from build123d import *

# Parameters (mm, degrees)
SKETCH2_R           = 0.75
BOSS_EXTRUDE1_DEPTH = 0.75
SKETCH3_R           = 0.375
BOSS_EXTRUDE2_DEPTH = 0.25
SKETCH4_R           = 1.125
CUT_EXTRUDE1_DEPTH  = 0.15
SKETCH5_R           = 1.1
SKETCH5_R_2         = 0.575
BOSS_EXTRUDE3_DEPTH = 0.15
SKETCH6_R           = 0.375
BOSS_EXTRUDE4_DEPTH = 0.25
SKETCH7_R           = 1.25
CUT_EXTRUDE2_DEPTH  = 5


with BuildPart() as part:
    # Sketch1 → Revolve1 (revolve)
    with BuildSketch(Plane.XY, mode=Mode.PRIVATE) as revolve1_sk:
        Polygon((0, 9.375), (-6.807, 9.375), (-6.807, 8.5), (-5.307, 8.5), (-5.307, 8.125), (-2.907, 8.125), (-2.907, 4.5), (-3.807, 4.5), (-3.807, 3.25), (-4.557, 3.25), (-4.557, 0), (4.557, 0), (4.557, 3.625), (4.057, 3.625), (4.057, 5), (0.943, 5), (0.943, 8.125), (4.193, 8.125), (4.193, 9), (6.193, 9), (6.193, 10), (6.693, 10), (6.693, 10.5), (5.593, 10.5), (5.593, 9.375), align=None)
    revolve(revolve1_sk.sketch.rotate(Axis((-4.557, 0, 0), (1, 0, 0)), 180), axis=Axis((-4.557, 0, 0), (1, 0, 0)))

    # Sketch2 → Boss-Extrude1 (add)
    with BuildSketch(Plane(origin=(0.943, 0, 0), x_dir=(0, 0, -1), z_dir=(1, 0, 0))):
        with Locations(Location((0, 6.25, 0), (0, 0, 270))):
            Circle(SKETCH2_R)
        with Locations(Location((3.125, 5.412658774, 0), (0, 0, 270))):
            Circle(SKETCH2_R)
        with Locations(Location((5.412658774, 3.125, 0), (0, 0, 270))):
            Circle(SKETCH2_R)
        with Locations(Location((6.25, 0, 0), (0, 0, 270))):
            Circle(SKETCH2_R)
        with Locations(Location((5.412658774, -3.125, 0), (0, 0, 270))):
            Circle(SKETCH2_R)
        with Locations(Location((3.125, -5.412658774, 0), (0, 0, 270))):
            Circle(SKETCH2_R)
        with Locations(Location((0, -6.25, 0), (0, 0, 270))):
            Circle(SKETCH2_R)
        with Locations(Location((-3.125, -5.412658774, 0), (0, 0, 270))):
            Circle(SKETCH2_R)
        with Locations(Location((-5.412658774, -3.125, 0), (0, 0, 270))):
            Circle(SKETCH2_R)
        with Locations(Location((-6.25, 0, 0), (0, 0, 270))):
            Circle(SKETCH2_R)
        with Locations(Location((-5.412658774, 3.125, 0), (0, 0, 270))):
            Circle(SKETCH2_R)
        with Locations(Location((-3.125, 5.412658774, 0), (0, 0, 270))):
            Circle(SKETCH2_R)
    extrude(amount=BOSS_EXTRUDE1_DEPTH)

    # Sketch3 → Boss-Extrude2 (add)
    with BuildSketch(Plane(origin=(4.057, 0, 0), x_dir=(0, 0, -1), z_dir=(1, 0, 0))):
        with Locations(Location((0, 4.25, 0), (0, 0, 270))):
            Circle(SKETCH3_R)
        with Locations(Location((2.125, 3.680607966, 0), (0, 0, 270))):
            Circle(SKETCH3_R)
        with Locations(Location((3.680607966, 2.125, 0), (0, 0, 270))):
            Circle(SKETCH3_R)
        with Locations(Location((4.25, 0, 0), (0, 0, 270))):
            Circle(SKETCH3_R)
        with Locations(Location((3.680607966, -2.125, 0), (0, 0, 270))):
            Circle(SKETCH3_R)
        with Locations(Location((2.125, -3.680607966, 0), (0, 0, 270))):
            Circle(SKETCH3_R)
        with Locations(Location((0, -4.25, 0), (0, 0, 270))):
            Circle(SKETCH3_R)
        with Locations(Location((-2.125, -3.680607966, 0), (0, 0, 270))):
            Circle(SKETCH3_R)
        with Locations(Location((-3.680607966, -2.125, 0), (0, 0, 270))):
            Circle(SKETCH3_R)
        with Locations(Location((-4.25, 0, 0), (0, 0, 270))):
            Circle(SKETCH3_R)
        with Locations(Location((-3.680607966, 2.125, 0), (0, 0, 270))):
            Circle(SKETCH3_R)
        with Locations(Location((-2.125, 3.680607966, 0), (0, 0, 270))):
            Circle(SKETCH3_R)
    extrude(amount=BOSS_EXTRUDE2_DEPTH)

    # Sketch4 → Cut-Extrude1 (cut)
    with BuildSketch(Plane(origin=(4.557, 0, 0), x_dir=(0, 0, -1), z_dir=(1, 0, 0))):
        with Locations(Location((0, 0, 0), (0, 0, 90))):
            Circle(SKETCH4_R)
    extrude(amount=-CUT_EXTRUDE1_DEPTH, mode=Mode.SUBTRACT)

    # Sketch5 → Boss-Extrude3 (add)
    # profile 1 of 3: a face of its own
    with BuildSketch(Plane(origin=(4.557, 0, 0), x_dir=(0, 0, -1), z_dir=(1, 0, 0))):
        with Locations(Location((0, 2.375, 0), (0, 0, 270))):
            Circle(SKETCH5_R)
        with Locations(Location((0, 2.375, 0), (0, 0, 90))):
            Circle(SKETCH5_R_2, mode=Mode.SUBTRACT)
    # profile 2 of 3: a face of its own
    with BuildSketch(Plane(origin=(4.557, 0, 0), x_dir=(0, 0, -1), z_dir=(1, 0, 0))):
        with Locations(Location((2.056810334, -1.1875, 0), (0, 0, 270))):
            Circle(SKETCH5_R)
        with Locations(Location((2.056810334, -1.1875, 0), (0, 0, 90))):
            Circle(SKETCH5_R_2, mode=Mode.SUBTRACT)
    # profile 3 of 3: a face of its own
    with BuildSketch(Plane(origin=(4.557, 0, 0), x_dir=(0, 0, -1), z_dir=(1, 0, 0))):
        with Locations(Location((-2.056810334, -1.1875, 0), (0, 0, 270))):
            Circle(SKETCH5_R)
        with Locations(Location((-2.056810334, -1.1875, 0), (0, 0, 90))):
            Circle(SKETCH5_R_2, mode=Mode.SUBTRACT)
    extrude(amount=BOSS_EXTRUDE3_DEPTH)

    # Sketch6 → Boss-Extrude4 (add)
    with BuildSketch(Plane.ZY.offset(3.807)):
        with Locations(Location((0, 3.81, 0), (0, 0, 90))):
            Circle(SKETCH6_R)
        with Locations(Location((1.905, 3.299556788, 0), (0, 0, 90))):
            Circle(SKETCH6_R)
        with Locations(Location((3.299556788, 1.905, 0), (0, 0, 90))):
            Circle(SKETCH6_R)
        with Locations(Location((3.81, 0, 0), (0, 0, 90))):
            Circle(SKETCH6_R)
        with Locations(Location((3.299556788, -1.905, 0), (0, 0, 90))):
            Circle(SKETCH6_R)
        with Locations(Location((1.905, -3.299556788, 0), (0, 0, 90))):
            Circle(SKETCH6_R)
        with Locations(Location((0, -3.81, 0), (0, 0, 90))):
            Circle(SKETCH6_R)
        with Locations(Location((-1.905, -3.299556788, 0), (0, 0, 90))):
            Circle(SKETCH6_R)
        with Locations(Location((-3.299556788, -1.905, 0), (0, 0, 90))):
            Circle(SKETCH6_R)
        with Locations(Location((-3.81, 0, 0), (0, 0, 90))):
            Circle(SKETCH6_R)
        with Locations(Location((-3.299556788, 1.905, 0), (0, 0, 90))):
            Circle(SKETCH6_R)
        with Locations(Location((-1.905, 3.299556788, 0), (0, 0, 90))):
            Circle(SKETCH6_R)
    extrude(amount=BOSS_EXTRUDE4_DEPTH)

    # Sketch7 → Cut-Extrude2 (cut)
    with BuildSketch(Plane.ZY.offset(4.557)):
        with Locations(Location((0, 0, 0), (0, 0, 270))):
            Circle(SKETCH7_R)
    extrude(amount=-CUT_EXTRUDE2_DEPTH, mode=Mode.SUBTRACT)


solid = part.part
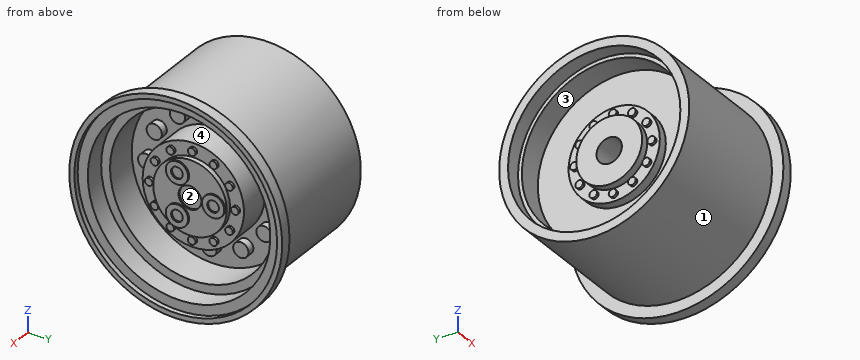
Can you work these out from the model? Positions are in its coordinate system, mm. Face numbers are marked on the shaded views. A direction names the side the tool comes from. Give positions to 0.01 mm unless a question says otherwise; leave off trailing zeros. Loops run counter-clockwise (first coordinate to the right, second up) from the corner with the lowest first, then second, coordinate; pieces in that order, holes last. Notation, with made-up numbers: (5, 76.25) -> (43, 76.25) arc R9 ccw to (43, 87.25) -> close; hole circle Ø6 at (78, -25.75). An arc over 180 degrees is marked (long way). Return JSON: item names as keys, results as strings.
Q1. On a 3-axis mill with a long thin cutter (end or side, diameter ignored), from which of +Z, -Z, +X, -X, +Y, -Y can I reach the whole of each face in a straight line? I mean the marked faces 3 and 4. Say none if no direction works.
Checks:
{"face 3": "-X", "face 4": "+X"}
Q2. I want a section at A-A, the plane x = 3.25. List the corners of the cut face in (y, z) for me (3 decimals), then the cut area to 3 significant figures.
Checks:
{"outline": "circle Ø18.75 at (0, 0); circle Ø10 at (0, 0); hole circle Ø16.25 at (0, 0)", "area": "147 mm2"}
Q3. For pin 1 Ø1.5 at (y, z) = (-2, 0) entering from -X; pin 2 Ø0.8 at (y, z) = (-4, 0) entering from -X; pin 3 Ø0.8 at (y, z) = (0.5, 6.5) entering from +X; pin 4 Ø6 at (y, z) = (6.5, -7) entering from +X, each with a flat end and sliding along its axis, tell me the tip position at first contact or that it passes through.
Checks:
{"pin 1": "stops at x = -4.56", "pin 2": "stops at x = -4.06", "pin 3": "stops at x = 1.69", "pin 4": "stops at x = 6.69"}
Q4. I want a section at B-B, the plane x = -0.75. List the corners of the cut face in (y, z) for me (3 decimals).
Checks:
{"outline": "circle Ø18.75 at (0, 0); hole circle Ø2.5 at (0, 0)"}
Q5. I need wall thicknesses on probe 1 along Y at (x, z) = (3, -0.25); probe 2 along Z at (x, y) = (-3.5, 0) (3 decimals); probe 3 along Y at (x, z) = (1.25, 1.5). Which ranges of each line are inside material? Lowest first, please.
Checks:
{"probe 1": "y = -9.37 to -8.12, -4.99 to 4.99, 8.12 to 9.37", "probe 2": "z = -9.375 to -8.125, -4.5 to -1.25, 1.25 to 4.5, 8.125 to 9.375", "probe 3": "y = -9.25 to -7.99, -4.77 to 4.77, 7.99 to 9.25"}
Q6. We'd pull the mould along Y, two halves only. Please class the marked faces 1 and 2: released by +Y, released by -Y, zero draft, split by the parting line, or undercut.
Checks:
{"face 1": "split by the parting line", "face 2": "undercut"}
Q7. I want a section at C-C, the plane z = 7.75. List the corners of the cut face in (x, y) for me.
Checks:
{"outline": "(-6.81, -5.28) -> (5.59, -5.28) -> (5.59, -7.08) -> (6.69, -7.08) -> (6.69, -6.32) -> (6.19, -6.32) -> (6.19, -4.58) -> (4.19, -4.58) -> (4.19, -2.44) -> (0.94, -2.44) -> (0.94, 2.44) -> (4.19, 2.44) -> (4.19, 4.58) -> (6.19, 4.58) -> (6.19, 6.32) -> (6.69, 6.32) -> (6.69, 7.08) -> (5.59, 7.08) -> (5.59, 5.28) -> (-6.81, 5.28) -> (-6.81, 3.49) -> (-5.31, 3.49) -> (-5.31, 2.44) -> (-2.91, 2.44) -> (-2.91, -2.44) -> (-5.31, -2.44) -> (-5.31, -3.49) -> (-6.81, -3.49) -> close"}
